Autodesk Inventor part; units mm, degrees
ref_plane "YZ Plane" through (0, 0, 0) normal (1, 0, 0) x (0, 1, 0)
ref_plane "XZ Plane" through (0, 0, 0) normal (0, 1, 0) x (-1, 0, 0)
ref_plane "XY Plane" through (0, 0, 0) normal (0, 0, 1) x (1, 0, 0)
sketch "Sketch1" plane through (0, 0, 0) normal (0, 0, 1) x (1, 0, 0)
  line L0 (20.828, 60.2998) -> (-20.828, 60.2998) construction
  line L1 (-38.1, 60.2998) -> (-38.1, 136.4998) construction
  line L2 (-38.1, 136.4998) -> (-20.828, 136.4998) construction
  line L3 (38.1, 136.4998) -> (-38.1, 136.4998) construction
  line L4 (37.846, 60.2998) -> (37.846, 136.4998) construction
  line L5 (-20.828, 47.6808) -> (-38.1, 47.6808) construction
  line L6 (-38.1, 136.4998) -> (37.846, 136.4998)
  line L7 (37.846, 136.4998) -> (37.846, 225.3188)
  line L8 (37.846, 225.3188) -> (-38.1, 225.3188)
  line L9 (-38.1, 225.3188) -> (-38.1, 136.4998)
  point P0 (0, 0)
extrude "Extrusion1" add sketch "Sketch1" along normal blind 8
sketch "Sketch2" plane through (0, 0, 0) normal (0, 0, -1) x (-1, 0, 0)
  line L0 (-37.846, 136.4998) -> (-37.846, 225.3188)
  line L1 (38.1, 225.3188) -> (38.1, 136.4998)
  line L2 (-37.846, 225.3188) -> (38.1, 225.3188)
  line L3 (38.1, 225.3188) -> (38.1, 215.3188)
  line L4 (38.1, 215.3188) -> (-37.846, 215.3188)
  line L5 (-37.846, 215.3188) -> (-37.846, 225.3188)
  point P0 (0, 0)
  dimension "d2" = 10
extrude "Extrusion2" add sketch "Sketch2" along normal blind 38
properties part number "MountingBracket"
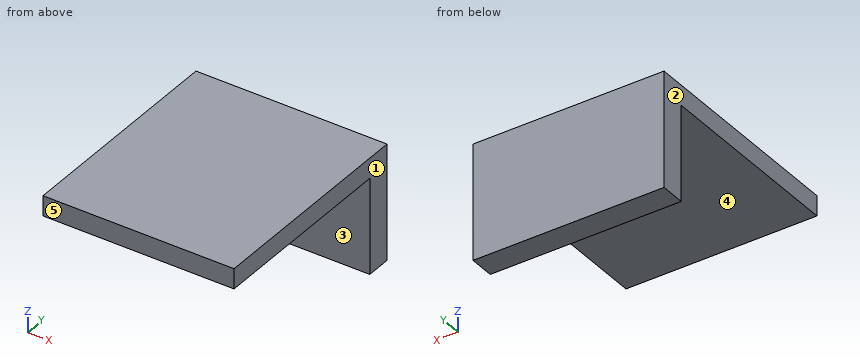
CAD build for the part. Positions are in the model's coordinates, mm. Face numbers are marked on the shaded views. A direction names the side the tool comes from. Coordinates: 2 decimals unless noted, no trailing zeros. Order: outer loops, then holes, each group sorted by start corner. A loop starts at its lowest first (then second) coordinate and runs counter-clockwise, first axis right, second up.
Item 1: Two-plate mould, pull along X, no slides. Class the marked faces 1, 2 and 3: +X half, -X half, draft (parallel to the pull), parting line (faces both ways), or undercut.
Check sheet entries:
face 1: +X half
face 2: -X half
face 3: draft
Item 2: Band-saw the part on B-B on y = 195.5. List the corners of the cut face in (x, z), plus the area to 3 significant figures.
Check sheet entries:
outline: (-38.1, 0) - (37.85, 0) - (37.85, 8) - (-38.1, 8) - close
area: 608 mm2
Item 3: Pin check, flat tips, straight feed: pin 1 Ø1.5 at (x, y) = (-11, 195.5) entering from -Z; pin 2 Ø3 at (x, z) = (-17, -3.5) entering from -Y. Stop position of each tip, or through.
Check sheet entries:
pin 1: stops at z = 0
pin 2: stops at y = 215.32
Item 4: Drill centre lines: L1, parallel to Y at x = -19, z = -15; L2, parallel to Z at x = 20.5, y = 195.5. Where is each one in solid material? Low to high.
Check sheet entries:
L1: y = 215.32 to 225.32
L2: z = 0 to 8
Item 5: 3-axis set-ups, long thin cutter, end or side, ignore diameter. For the marked faces 4 and 5: which of +Z, -Z, +X, -X, +Y, -Y reach the whole face in a straight line?
Check sheet entries:
face 4: -Z, +X, -X, -Y
face 5: +Z, -Z, +X, -X, -Y
Item 6: Band-saw the part on C-C on z = -30.5. List the corners of the cut face in (x, y), plus the area to 3 significant figures.
Check sheet entries:
outline: (-38.1, 215.32) - (37.85, 215.32) - (37.85, 225.32) - (-38.1, 225.32) - close
area: 759 mm2
Item 7: Band-saw the part on A-A on x = 12. List the corners of the cut face in (y, z).
Check sheet entries:
outline: (136.5, 0) - (215.32, 0) - (215.32, -38) - (225.32, -38) - (225.32, 8) - (136.5, 8) - close
